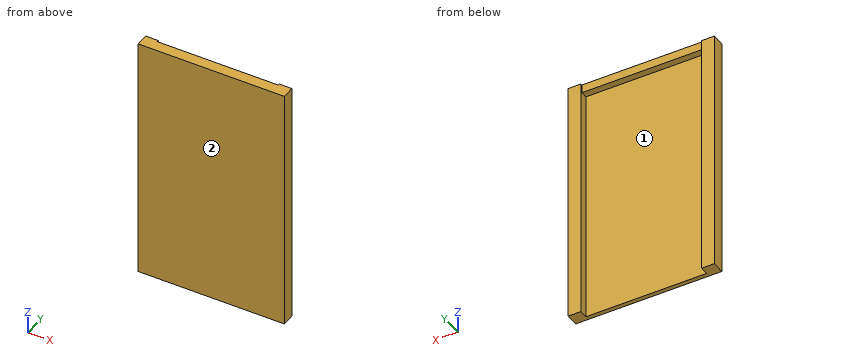
```python
from build123d import *

# Parameters (mm, degrees)
BOSS_EXTRUDE1_DEPTH = 2.6
SKETCH3_W           = 3
SKETCH3_H           = 59.15
BOSS_EXTRUDE2_DEPTH = 0.4
SKETCH5_W           = 28.5
SKETCH5_H           = 1
BOSS_EXTRUDE3_DEPTH = 57.15


with BuildPart() as part:
    # Sketch1 → Boss-Extrude1 (new body)
    with BuildSketch(Plane(origin=(0, 0, 0), x_dir=(1, 0, 0), z_dir=(0, 1, 0))):
        Polygon((0, 0), (17.25, 0), (17.25, 59.15), (14.25, 59.15), (14.25, 2), (0, 2), align=None)
    boss_extrude1 = extrude(amount=BOSS_EXTRUDE1_DEPTH)

    # Sketch3 → Boss-Extrude2 (add)
    with BuildSketch(Plane(origin=(0, 2.6, 0), x_dir=(1, 0, 0), z_dir=(0, 1, 0))):
        with Locations((15.75, 29.575)):
            Rectangle(SKETCH3_W, SKETCH3_H)
    boss_extrude2 = extrude(amount=BOSS_EXTRUDE2_DEPTH)

    # Mirror2: Boss-Extrude1, Boss-Extrude2 across plane
    add(boss_extrude1.mirror(Plane(origin=(0, 0, 0), x_dir=(0, 0, 1), z_dir=(1, 0, 0))))
    add(boss_extrude2.mirror(Plane(origin=(0, 0, 0), x_dir=(0, 0, 1), z_dir=(1, 0, 0))))

    # Sketch5 → Boss-Extrude3 (add, through all)
    with BuildSketch(Plane(origin=(0, 0, -2), x_dir=(-1, 0, 0), z_dir=(0, 0, -1))):
        with Locations((0, 0.5)):
            Rectangle(SKETCH5_W, SKETCH5_H)
    extrude(amount=BOSS_EXTRUDE3_DEPTH)


solid = part.part
```
Part model, mm, in its own coordinate system. Face numbers are marked on the shaded views. A direction names the side the tool comes from. Give positions to 0.01 mm unless a question says otherwise; leave off trailing zeros. Order: outer loops, then holes, each group sorted by start corner. A loop starts at its lowest first (then second) coordinate and runs counter-clockwise, first axis right, second up. Notation, with made-up numbers: M 44.5,-25 L 98.5,-25 A14 cw 98.5,-5 Z; hole C -8,65 d8. An arc over 180 degrees is marked long. Use a Markdown table: item, result. Add a question column.
(1) Saw through at A-A, the plane z = -14. Give the cut face in (x, y), and give its area (3 significant figures).
(2) 3-axis set-ups, long thin cutter, end or side, ignore diameter. For the marked faces 1 and 2: which of +Z, -Z, +X, -X, +Y, -Y reach the whole face in a straight line?
(3) Saw through at B-B, the plane y = 2. Give the cut face in (x, z), and give its area (3 significant figures).
(4) Saw through at C-C, the plane x = -13. Give the cut face in (y, z).
(5) Drop flat-ended pins along their axis: P1, Ø8.5, axis at x = 5.5, z = -21, coming from the +Y side; P2, Ø1, axis at x = -0.5, z = -1, coming from the +Y side. Give the stop position or say it passes through.
(6) Probe line 1 along X through (y, z) = (1.1, -7); line 2 along Y through (x, z) = (9.5, -29); line 3 along Z through (x, y) = (-10, 2.3). List the from-to ranges inside material, lowest first. Write a range as [from, to].
Answer key:
| question | item | result |
|---|---|---|
| 1 | outline | M -17.25,0 L 17.25,0 L 17.25,3 L 14.25,3 L 14.25,1 L -14.25,1 L -14.25,3 L -17.25,3 Z |
| 1 | area | 46.5 mm^2 |
| 2 | face 1 | -Z, +Y |
| 2 | face 2 | +Z, -Z, +X, -X, -Y |
| 3 | outline | M -17.25,-59.15 L -14.25,-59.15 L -14.25,-2 L 14.25,-2 L 14.25,-59.15 L 17.25,-59.15 L 17.25,0 L -17.25,0 Z |
| 3 | area | 412 mm^2 |
| 4 | outline | M 0,-59.15 L 1,-59.15 L 1,-2 L 2.6,-2 L 2.6,0 L 0,0 Z |
| 5 | P1 | y = 1 |
| 5 | P2 | y = 2.6 |
| 6 | line 1 | [-17.25, -14.25], [14.25, 17.25] |
| 6 | line 2 | [0, 1] |
| 6 | line 3 | [-2, 0] |
